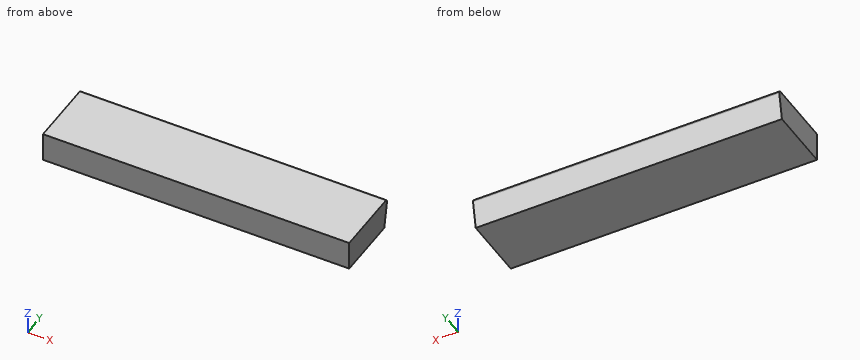
Autodesk Inventor part; units mm, degrees
ref_plane "YZ Plane" through (0, 0, 0) normal (1, 0, 0) x (0, 1, 0)
ref_plane "XZ Plane" through (0, 0, 0) normal (0, 1, 0) x (-1, 0, 0)
ref_plane "XY Plane" through (0, 0, 0) normal (0, 0, 1) x (1, 0, 0)
sketch "Sketch2" plane through (0, 0, 0) normal (1, 0, 0) x (0, 1, 0)
  line L0 (0, 0) -> (0, 152.4)
  line L1 (0, 152.4) -> (342.9, 152.4)
  line L2 (0, 0) -> (330.2, 0)
  line L3 (330.2, 0) -> (355.3918, 137.4098)
  arc A0 (355.3918, 137.4098) -> (342.9, 152.4) centre (342.9, 139.7) ccw
  point P0 (358.14, 152.4)
  dimension "d2" = 152.4
  dimension "d3" = 330.2
  dimension "d4" = 12.7
  dimension "d7" = 342.9
extrude "Extrusion1" add sketch "Sketch2" along normal blind 1595.12
properties part number "B" material "Granite, Cut, Polished"
Here's how the part is built. I have some questions about the finished solid (model axes, mm). Coordinates: 2 decimals unless noted, no trailing zeros. Loops run counter-clockwise (first coordinate to the right, second up) from the corner with the lowest first, then second, coordinate; pieces in that order, holes last.
1. Imagine slicing it at A-A, the plane x = 110.5. Please give me the cut outline in (y, z), and give its area (3 significant figures).
2. I need wall thicknesses on L1, parallel to Y at x = 798, z = 68; L2, parallel to Y at x = 1143.5, z = 99. Which ranges of each line are inside material? Lowest first, please.
3. Imagine slicing it at B-B, the plane z = 20. Please give me the cut outline in (x, y), and give its area (3 significant figures).
4. For P1, Ø2, axis at x = 671.5, y = 308, coming from the -Z side, with a flat end and sliding along its axis, tell me the tip position at first contact or that it passes through.
Taken from the geometry:
1. outline: (0, 0) - (330.2, 0) - (355.39, 137.41) arc R12.7 ccw to (342.9, 152.4) - (0, 152.4) - close
1. area: 52,400 mm2
2. L1: y = 0 to 342.67
2. L2: y = 0 to 348.35
3. outline: (0, 0) - (1595.12, 0) - (1595.12, 333.87) - (0, 333.87) - close
3. area: 533,000 mm2
4. P1: stops at z = 0
